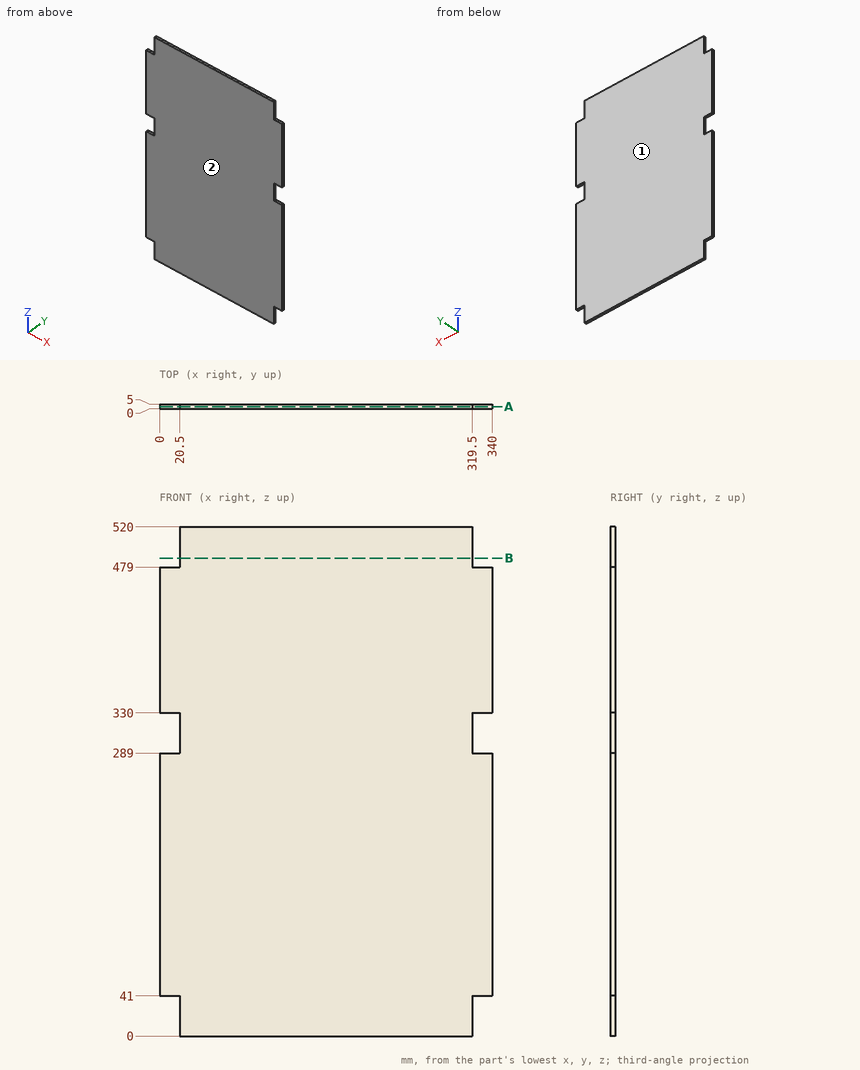
The figure shows three views and two pictorial views of one solid part (mm, origin at its lowest corner). Answer the questions. Round coordinates to 2 decimals unless told otherwise and drop trailing zeros. Write each loop counter-clockwise with the first axis right and the second up, starting at its lowest first coordinate (ties: lowest second). Pieces come first, ordered by that corner, then holes. Notation, with made-up numbers: (-30.75, 4) - (5.25, 4) arc R16 ccw to (5.25, 26) - close; hole circle Ø11 at (45, 35). An arc over 180 degrees is marked (long way). Answer in a Markdown table with one row per item. Add a question column.
1. Find the intervals of material crossed by line 1 along Z through (x, y) = (17, 1.2); line 2 along X through (y, z) = (2, 325.5), in increasing order. Write a range as from..to.
2. A cutting plane is placed at A-A, the plane y = 2.4. Determine the outline of the cut face in (x, z).
3. Given pin 1 (1.5 mm diameter, centred on x = 7.5, y = 2, fed in from +Z); pin 2 (2.5 mm diameter, centred on x = 327.5, y = 2, fed in from -Z); pin 3 (1.5 mm diameter, centred on y = 2.5, z = 495.5, fed in from +X), each flat-ended and moving along its own axis, determine where each tip first touches the part or whether it passes through.
4. The mould has two halves that part along Y. Classify the marked faces 1 and 2: +Y half, -Y half, draft (parallel to the pull), parting line (faces both ways), or undercut.
5. A cutting plane is placed at B-B, the plane z = 488. Determine the outline of the cut face in (x, y).
Worked out:
| question | item | result |
|---|---|---|
| 1 | line 1 | 41..289, 330..479 |
| 1 | line 2 | 20.5..319.5 |
| 2 | outline | (0, 41) - (20.5, 41) - (20.5, 0) - (319.5, 0) - (319.5, 41) - (340, 41) - (340, 289) - (319.5, 289) - (319.5, 330) - (340, 330) - (340, 479) - (319.5, 479) - (319.5, 520) - (20.5, 520) - (20.5, 479) - (0, 479) - (0, 330) - (20.5, 330) - (20.5, 289) - (0, 289) - close |
| 3 | pin 1 | z = 479 |
| 3 | pin 2 | z = 41 |
| 3 | pin 3 | x = 319.5 |
| 4 | face 1 | +Y half |
| 4 | face 2 | -Y half |
| 5 | outline | (20.5, 0) - (319.5, 0) - (319.5, 5) - (20.5, 5) - close |
